CAD build for the part. Positions are in the model's coordinates, mm. Round coordinates to 2 decimals unless told otherwise and drop trailing zeros. Loops run counter-clockwise (first coordinate to the right, second up) from the corner with the lowest first, then second, coordinate; pieces in that order, holes last.
Autodesk Inventor part; units mm, degrees
ref_plane "YZ Plane" through (0, 0, 0) normal (1, 0, 0) x (0, 1, 0)
ref_plane "XZ Plane" through (0, 0, 0) normal (0, 1, 0) x (-1, 0, 0)
ref_plane "XY Plane" through (0, 0, 0) normal (0, 0, 1) x (1, 0, 0)
sketch "Sketch1" plane through (0, 0, 0) normal (0, 1, 0) x (-1, 0, 0)
  line L0 (0, 0) -> (200, 0)
  line L1 (200, 0) -> (200, -200)
  line L2 (200, -200) -> (0, -200)
  line L3 (0, -200) -> (0, 0)
  circle A0 centre (100, -100) radius 92.5
  dimension "d0" = 200
  dimension "d1" = 200
  dimension "d2" = 185
extrude "Extrusion1" add sketch "Sketch1" against normal blind 1.5
sketch "Sketch3" plane through (0, -1.5, 0) normal (0, -1, 0) x (1, 0, 0)
  line L0 (-197.5, -2.5) -> (-2.5, -2.5)
  line L1 (-2.5, -2.5) -> (-2.5, -197.5)
  line L2 (-2.5, -197.5) -> (-197.5, -197.5)
  line L3 (-197.5, -197.5) -> (-197.5, -2.5)
  circle A0 centre (-100, -100) radius 87
  dimension "d5" = 195
  dimension "d6" = 195
  dimension "d7" = 174
  dimension "d11" = 0
extrude "Extrusion2" add sketch "Sketch3" along normal blind 2
properties part number "box cover"
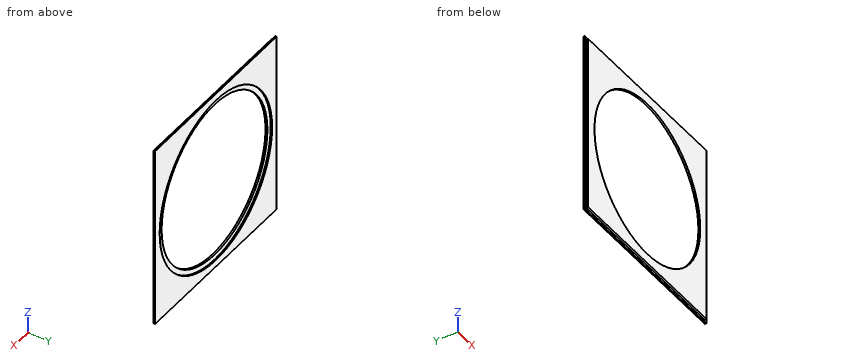
Item 1: Cut at A-A (z = -100). List the corners of the cut face in (x, y), plus the area to 3 significant figures.
Verdict:
outline: (-200, -1.5) - (-197.5, -1.5) - (-197.5, -3.5) - (-187, -3.5) - (-187, -1.5) - (-192.5, -1.5) - (-192.5, 0) - (-200, 0) - close; (-13, -3.5) - (-2.5, -3.5) - (-2.5, -1.5) - (0, -1.5) - (0, 0) - (-7.5, 0) - (-7.5, -1.5) - (-13, -1.5) - close
area: 64.5 mm2
Item 2: Wall check: L1, parallel to Z at x = -100, y = -0.5; L2, parallel to Y at x = -53, z = -21; L3, parallel to Z at x = -100, y = -3.1. Give the ranges that are in metal, low to high.
Verdict:
L1: z = -200 to -192.5, -7.5 to 0
L2: y = -3.5 to -1.5
L3: z = -197.5 to -187, -13 to -2.5
Item 3: Flat gauge pins, fed straight in: P1, Ø1, axis at y = -2.5, z = -99, coming from the +X side; P2, Ø1, axis at y = -3, z = -114.5, coming from the -X side; P3, Ø1.6, axis at x = -79.5, y = -2.5, coming from the +Z side. Where does each tip first touch, or does it go through?
Verdict:
P1: stops at x = -2.5
P2: stops at x = -197.5
P3: stops at z = -2.5
Item 4: Cut at C-C (y = -2.65). List the corners of the cut face in (x, z).
Verdict:
outline: (-197.5, -197.5) - (-2.5, -197.5) - (-2.5, -2.5) - (-197.5, -2.5) - close; hole circle Ø174 at (-100, -100)
Item 5: Cut at B-B (x = -100). List the corners of the cut face in (y, z).
Verdict:
outline: (-3.5, -197.5) - (-1.5, -197.5) - (-1.5, -200) - (0, -200) - (0, -192.5) - (-1.5, -192.5) - (-1.5, -187) - (-3.5, -187) - close; (-3.5, -13) - (-1.5, -13) - (-1.5, -7.5) - (0, -7.5) - (0, 0) - (-1.5, 0) - (-1.5, -2.5) - (-3.5, -2.5) - close
